Autodesk Inventor part; units mm, degrees
ref_plane "YZ Plane" through (0, 0, 0) normal (1, 0, 0) x (0, 1, 0)
ref_plane "XZ Plane" through (0, 0, 0) normal (0, 1, 0) x (-1, 0, 0)
ref_plane "XY Plane" through (0, 0, 0) normal (0, 0, 1) x (1, 0, 0)
sketch "BASEsc" plane through (0, 0, 0) normal (0, 1, 0) x (-1, 0, 0)
  point P0 (0, 0)
sketch "スケッチ2" plane through (0, 0, 0) normal (0, 1, 0) x (-1, 0, 0)
  circle A0 centre (0, 0) radius 17.4
  line L0 (0, -17.4) -> (0, -15.4)
  line L1 (2.75, -16.847) -> (-2.75, -16.847) construction
  line L2 (-2.75, -16.847) -> (-2.75, -17.953) construction
  line L3 (-2.75, -17.953) -> (2.75, -17.953) construction
  line L4 (2.75, -17.953) -> (2.75, -16.847) construction
  line L5 (2.75, -16.847) -> (-2.75, -17.953) construction
  line L6 (-2.75, -16.847) -> (2.75, -17.953) construction
  arc A1 (2.75, -17.1813) -> (-2.75, -17.1813) centre (0, -18.4134) ccw
  arc A2 (16.2545, -6.2091) -> (13.5045, -10.9722) centre (15.9465, -9.2067) ccw
  arc A3 (13.5045, 10.9722) -> (16.2545, 6.2091) centre (15.9465, 9.2067) ccw
  arc A4 (-2.75, 17.1813) -> (2.75, 17.1813) centre (0, 18.4134) ccw
  arc A5 (-16.2545, 6.2091) -> (-13.5045, 10.9722) centre (-15.9465, 9.2067) ccw
  arc A6 (-13.5045, -10.9722) -> (-16.2545, -6.2091) centre (-15.9465, -9.2067) ccw
  circle A7 centre (0, 0) radius 19.25
  point P0 (13.3368, -7.7)
  point P1 (13.3368, 7.7)
  point P2 (0, 15.4)
  point P3 (-13.3368, 7.7)
  point P4 (-13.3368, -7.7)
  point P5 (13.5045, -10.9722)
  point P6 (-13.5045, -10.9722)
  point P7 (-16.2545, -6.2091)
  point P8 (-13.5045, 10.9722)
  point P9 (16.2545, 6.2091)
  dimension "d0" = 34.8
  dimension "d1" = 2
  dimension "d2" = 5.5
  dimension "d5" = 360
  dimension "d7" = 38.5
extrude "押し出し1" add sketch "スケッチ2" along normal blind 2.5 contours A3 A0 | A0 A2 | A4 A0 | A0 L0 A1 | A0 A1 L0 | A5 A0 | A0 A6 | A7
equation "\"BendRadius\" = Thickness"
equation "\"BendReliefWidth\" = Thickness"
equation "\"BendReliefDepth\" = 0.5 * Thickness"
equation "\"CornerReliefSize\" = 4 * Thickness"
equation "\"MinimumRemnant\" = 2 * Thickness"
equation "\"TransitionRadius\" = BendRadius"
equation "\"JacobiRadiusSize\" = BendRadius"
equation "\"GapSize\" = Thickness"
properties part number "template"
Here's how the part is built. I have some questions about the finished solid (model axes, mm). A direction names the side the tool comes from. Round coordinates to 2 decimals unless told otherwise and drop trailing zeros. Loops run counter-clockwise (first coordinate to the right, second up) from the corner with the lowest first, then second, coordinate; pieces in that order, holes last. Notation, with made-up numbers: (63.25, 83.5) -> (100.25, 83.5) arc R20 ccw to (100.25, 99.5) -> close; hole circle Ø10 at (29, 49). An arc over 180 degrees is marked (long way). Write each question's results on one line, items separated by ' | '.
(1) For faces 1 (the face through (0, 2.5, 16)), 2 (the face through (-13.313, 1.232, -7.742)), which set-ups out of +Z, -Z, +X, -X, +Y, -Y let a thin tool reach every point of the face, with its end or its side?
Worked answers:
face 1: +Z, -Z, +X, -X, +Y | face 2: +Y, -Y
(2) If we section it at A-A, the plane x = 0: List the corners of the cut face in (y, z) for me, then the cut area to 4 significant figures.
Worked answers:
outline: (0, -19.25) -> (2.5, -19.25) -> (2.5, -15.4) -> (0, -15.4) -> close; (0, 15.4) -> (2.5, 15.4) -> (2.5, 19.25) -> (0, 19.25) -> close | area: 19.25 mm2
(3) For P1, Ø1, axis at y = 1.5, z = -3.5, coming from the -X side; P2, Ø1.5, axis at y = 0.5, z = -12, coming from the -X side, each with a flat end and sliding along its axis, tell me the tip position at first contact or that it passes through.
Worked answers:
P1: x = -19.01 | P2: x = -15.62
(4) If I drill on L1, parallel to X at y = 0.7, z = -0.5; L2, parallel to X at y = 2.3, z = 4.5; L3, parallel to Z at x = -11, y = 1.5, over which ranges is the centre line in solid material (lowest first)?
Worked answers:
L1: -19.24 to -17.39, 17.39 to 19.24 | L2: -18.72 to -16.81, 16.81 to 18.72 | L3: -15.8 to -13.48, 13.48 to 15.8
(5) If we section it at B-B, the plane z = 0: List the corners of the cut face in (x, y) for me, then the cut area to 3 significant figures.
Worked answers:
outline: (-19.25, 0) -> (-17.4, 0) -> (-17.4, 2.5) -> (-19.25, 2.5) -> close; (17.4, 0) -> (19.25, 0) -> (19.25, 2.5) -> (17.4, 2.5) -> close | area: 9.25 mm2
(6) If we section it at C-C, the plane y = 1.1: List the corners of the cut face in (x, z) for me.
Worked answers:
outline: circle Ø38.5 at (0, 0); hole (-16.25, -6.21) arc R3.01 cw to (-13.5, -10.97) arc R17.4 ccw to (-2.75, -17.18) arc R3.01 cw to (2.75, -17.18) arc R17.4 ccw to (13.5, -10.97) arc R3.01 cw to (16.25, -6.21) arc R17.4 ccw to (16.25, 6.21) arc R3.01 cw to (13.5, 10.97) arc R17.4 ccw to (2.75, 17.18) arc R3.01 cw to (-2.75, 17.18) arc R17.4 ccw to (-13.5, 10.97) arc R3.01 cw to (-16.25, 6.21) arc R17.4 ccw to start
(7) We'd pull the mould along X, two halves only. Please class faces 3 (the face through (0, 1.2, -15.4)), 4 (the face through (15.28, 1.23, 11.71)), 5 (the face through (0, 0, 16)): released by +X, released by -X, zero draft, split by the parting line, or undercut.
Worked answers:
face 3: undercut | face 4: split by the parting line | face 5: zero draft
